Read the model definition and answer for the solid it produces. Units are mm, in the model's axes. A direction names the side the tool comes from. Round coordinates to 2 decimals unless told otherwise and drop trailing zeros. Order: outer loops, then holes, each group sorted by start corner. A loop starts at its lowest first (then second) coordinate and runs counter-clockwise, first axis right, second up. Notation, with made-up numbers: M 47,-31 L 56,-31 A5 cw 56,-27 Z; hole C -39.5,32 d4. An arc over 180 degrees is marked long. Use one line per item in the form item = value. Start each with the question number.
from build123d import *

# Parameters (mm, degrees)
ESTRUSIONE_ESTRUSIONE1_DEPTH  = 22.5
SCHIZZO2_W                    = 45
SCHIZZO2_H                    = 73.192388155
ESTRUSIONE_ESTRUSIONE2_DEPTH  = 16
ESTRUSIONE_ESTRUSIONE3_DEPTH  = 13
TAGLIO_ESTRUSIONE1_DEPTH      = 1
TAGLIO_ESTRUSIONE1_DEPTH_BACK = 46
SCHIZZO5_R                    = 12.5
TAGLIO_ESTRUSIONE2_DEPTH      = 14
SCHIZZO6_R                    = 6.5
TAGLIO_ESTRUSIONE3_DEPTH      = 127.488852712
SCHIZZO7_R                    = 4
TAGLIO_ESTRUSIONE4_DEPTH      = 59.254833996


with BuildPart() as part:
    # Schizzo1 → Estrusione-Estrusione1 (new body, symmetric)
    with BuildSketch(Plane.XY):
        Polygon((-49, 13), (-49, 0), (49, 0), (94.254833996, -45.254833996), (100.754833996, -38.754833996), (49, 13), align=None)
    extrude(amount=ESTRUSIONE_ESTRUSIONE1_DEPTH, both=True)

    # Schizzo2 → Estrusione-Estrusione2 (add)
    with BuildSketch(Plane(origin=(31, 31, 0), x_dir=(0, 0, -1), z_dir=(0.707106781, 0.707106781, 0))):
        with Locations((0, -62.052038201)):
            Rectangle(SCHIZZO2_W, SCHIZZO2_H)
    extrude(amount=ESTRUSIONE_ESTRUSIONE2_DEPTH)

    # Schizzo3 → Estrusione-Estrusione3 (add)
    with BuildSketch(Plane.ZY.offset(49)):
        with BuildLine():
            Line((-22.5, 0), (-22.5, 26))
            ThreePointArc((-22.5, 26), (0, 48.5), (22.5, 26))
            Line((22.5, 26), (22.5, 0))
            Line((22.5, 0), (-22.5, 0))
        make_face()
    extrude(amount=-ESTRUSIONE_ESTRUSIONE3_DEPTH)

    # Schizzo4 → Taglio-Estrusione1 (cut, two sides)
    with BuildSketch(Plane.XY.offset(22.5)) as taglio_estrusione1_sk:
        Polygon((73.748737342, -24.748737342), (85.062445841, -13.435028843), (98.497474683, -26.870057685), (87.183766184, -38.183766184), align=None)
    extrude(amount=TAGLIO_ESTRUSIONE1_DEPTH, mode=Mode.SUBTRACT)
    extrude(taglio_estrusione1_sk.sketch, amount=-TAGLIO_ESTRUSIONE1_DEPTH_BACK, mode=Mode.SUBTRACT)

    # Schizzo5 → Taglio-Estrusione2 (cut, through all)
    with BuildSketch(Plane(origin=(-36, 0, 0), x_dir=(0, 0, -1), z_dir=(1, 0, 0))):
        with Locations((0, 26)):
            Circle(SCHIZZO5_R)
    extrude(amount=-TAGLIO_ESTRUSIONE2_DEPTH, mode=Mode.SUBTRACT)

    # Schizzo6 → Taglio-Estrusione3 (cut, through all)
    with BuildSketch(Plane(origin=(42.313708499, 42.313708499, 0), x_dir=(0, 0, -1), z_dir=(0.707106781, 0.707106781, 0))):
        with Locations((0, -79.648232278)):
            Circle(SCHIZZO6_R)
    extrude(amount=-TAGLIO_ESTRUSIONE3_DEPTH, mode=Mode.SUBTRACT)

    # Schizzo7 → Taglio-Estrusione4 (cut, through all)
    with BuildSketch(Plane(origin=(0, 13, 0), x_dir=(1, 0, 0), z_dir=(0, 1, 0))):
        with Locations((-23, 9.5)):
            Circle(SCHIZZO7_R)
        with Locations((31, 9.5)):
            Circle(SCHIZZO7_R)
    taglio_estrusione4 = extrude(amount=-TAGLIO_ESTRUSIONE4_DEPTH, mode=Mode.SUBTRACT)

    # Specchia1: Taglio-Estrusione4 across plane
    add(taglio_estrusione4.mirror(Plane.XY), mode=Mode.SUBTRACT)


solid = part.part
Item 1: Section D-D (x = 12) is taken. Write down the section's boundary in (y, z).
Item 2: Find the intervals of material crossed by L1, parallel to Z at x = -23, y = 9.25; L2, parallel to Y at x = -43.5, z = 0; L3, parallel to Y at x = 40, z = 19.5, in increasing order. Write a range as [from, to].
Item 3: A tool of negligible diameter and unlimited length cuts with its end or side. For faces 4 (the flat face through (55, 19, 0)), 5 (the flat face through (92.92, -32.45, 0.32)), 6 (the flat face through (79.3, -19.2, 0.3)), from which of +Z, -Z, +X, -X, +Y, -Y can it reach the whole face along a straight path? Write none if from no direction.
Item 4: Section A-A (x = 31) is taken. Write down the section's boundary in (y, z), and give its area (3 significant figures).
Item 5: For a pull along Y with two mould halves and no side action, classify faces 1 (the flat face through (-36, 39, 0)), 2 (the cylindrical face through (-42.41, 14.91, -5.77)), 3 (the flat face through (-1, 0, 0)) as pulls with the +Y half, pulls with the -Y half, needs draft (parallel to the pull), parting line crosses it, or undercut.
Item 6: Given P1, Ø3, axis at x = 84, z = 15, coming from the -Y side; P2, Ø1, axis at x = 43, z = -13, coming from the +Y side; P3, Ø18, axis at y = 36, z = 5.5, coming from the +X side, each flat-ended and moving along its own axis, determine where each tip first touches the part or whether it passes through.
Item 7: Section B-B (z = 9.5) is taken. Write down the section's boundary in (x, y), and give its area (3 significant figures).
Item 8: Section C-C (z = 0) is taken. Write down the section's boundary in (x, y), and give its area (3 significant figures).
The answers:
q1.outline = M 0,-22.5 L 13,-22.5 L 13,22.5 L 0,22.5 Z
q2.L1 = [-22.5, -13.5], [-5.5, 5.5], [13.5, 22.5]
q2.L2 = [0, 13.5], [38.5, 48.5]
q2.L3 = [0, 13]
q3.face_4 = +Z, -Z, +Y
q3.face_5 = +Z, -Z, -X
q3.face_6 = +Z, -Z, -Y
q4.outline = M 0,-22.5 L 13,-22.5 L 13,-13.5 L 0,-13.5 Z; M 0,-5.5 L 13,-5.5 L 13,5.5 L 0,5.5 Z; M 0,13.5 L 13,13.5 L 13,22.5 L 0,22.5 Z
q4.area = 377 mm²
q5.face_1 = needs draft
q5.face_2 = undercut
q5.face_3 = pulls with the -Y half
q6.P1 = -16
q6.P2 = 13
q6.P3 = -36
q7.outline = M -49,0 L -27,0 L -27,13 L -36,13 L -36,17.88 L -49,17.88 Z; M -49,34.12 L -36,34.12 L -36,46.4 L -49,46.4 Z; M -19,0 L 27,0 L 27,13 L -19,13 Z; M 35,0 L 49,0 L 73.75,-24.75 L 85.06,-13.44 L 98.5,-26.87 L 87.18,-38.18 L 94.25,-45.25 L 112.07,-27.44 L 60.31,24.31 L 49,13 L 35,13 Z
q7.area = 2,790 mm²
q8.outline = M -49,0 L 49,0 L 73.75,-24.75 L 85.06,-13.44 L 87.54,-15.91 L 94.04,-9.41 L 60.31,24.31 L 49,13 L -36,13 L -36,13.5 L -49,13.5 Z; M -49,38.5 L -36,38.5 L -36,48.5 L -49,48.5 Z; M 87.18,-38.18 L 94.25,-45.25 L 112.07,-27.44 L 103.23,-18.6 L 96.73,-25.1 L 98.5,-26.87 Z
q8.area = 2,790 mm²
